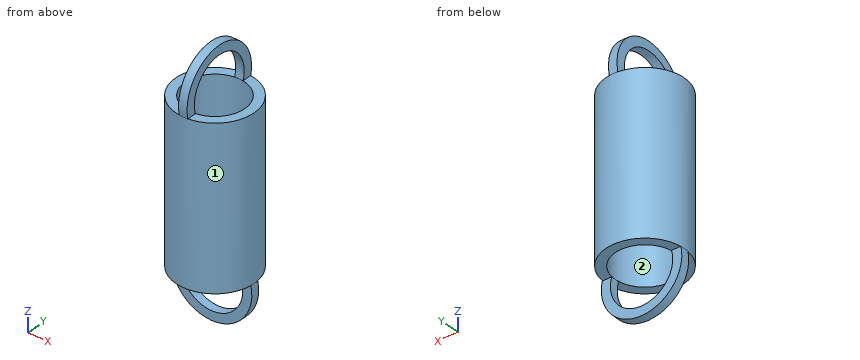
from build123d import *

# Parameters (mm, degrees)
SKETCH1_R           = 4.6
SKETCH1_R_2         = 3.5
BOSS_EXTRUDE1_DEPTH = 9.35
BOSS_EXTRUDE2_DEPTH = 0.5
BOSS_EXTRUDE3_DEPTH = 0.5


with BuildPart() as part:
    # Sketch1 → Boss-Extrude1 (new, symmetric)
    with BuildSketch(Plane.XY):
        Circle(SKETCH1_R)
        Circle(SKETCH1_R_2, mode=Mode.SUBTRACT)
    extrude(amount=BOSS_EXTRUDE1_DEPTH, both=True)

    # Sketch2 → Boss-Extrude2 (add, symmetric)
    with BuildSketch(Plane(origin=(0, 0, 0), x_dir=(0, 0, -1), z_dir=(1, 0, 0))):
        with BuildLine():
            Line((-9.35, -4.6), (-9.35, -3.5))
            ThreePointArc((-9.35, -3.5), (-13.990054945, 0), (-9.35, 3.5))
            Line((-9.35, 3.5), (-9.35, 4.6))
            ThreePointArc((-9.35, 4.6), (-15.057440918, 0), (-9.35, -4.6))
        make_face()
    extrude(amount=BOSS_EXTRUDE2_DEPTH, both=True)

    # Sketch4 → Boss-Extrude3 (add, symmetric)
    with BuildSketch(Plane(origin=(0, 0, 0), x_dir=(1, 0, 0), z_dir=(0, 1, 0))):
        with BuildLine():
            Line((4.6, 9.35), (3.5, 9.35))
            ThreePointArc((3.5, 9.35), (0, 13.990054945), (-3.5, 9.35))
            Line((-3.5, 9.35), (-4.6, 9.35))
            ThreePointArc((-4.6, 9.35), (0, 15.057440918), (4.6, 9.35))
        make_face()
    extrude(amount=BOSS_EXTRUDE3_DEPTH, both=True)


solid = part.part
For this review, take the finished solid that the model builds, in its own axes (mm). Face numbers are marked on the shaded views. Coordinates: 2 decimals unless noted, no trailing zeros. Loops run counter-clockwise (first coordinate to the right, second up) from the corner with the lowest first, then second, coordinate; pieces in that order, holes last. Notation, with made-up numbers: (18, 39) - (30, 39) arc R27 ccw to (30, 68) - close; hole circle Ø5 at (56.25, 60.25). An arc over 180 degrees is marked (long way). Use a Markdown table: item, result. Add a question column.
Item 1: We need section A-A (z = -10.35). Give the boundary of the cut face in (x, y), and give its area (3 significant figures).
Item 2: For line 1 (Z direction, x = 0, y = -0.1); line 2 (X direction, y = 0, z = -1.75); line 3 (Y direction, x = 0.2, z = 10.35), list the stretches that pass through material, from the lowest coordinate up.
Item 3: Insertion check: pin 1 Ø3 at (y, z) = (-2, -8.5) entering from -X; pin 2 Ø1.4 at (x, y) = (0, 1.5) entering from -Z; pin 3 Ø3 at (x, z) = (0, -13) entering from +Y; pin 4 Ø1.7 at (x, z) = (1, -11.5) entering from -Y. Each pin has a flat end and moves straight along its axis. Give the tip position at first contact, or say it passes through.
Item 4: We need section B-B (y = 1.75). Give the boundary of the cut face in (x, z), and give its area (3 significant figures).
Item 5: Mouldability with a two-part tool opening along X and no side actions: class the marked faces 1 and 2 as pulls with the +X half, pulls with the -X half, needs draft (parallel to the pull), parting line crosses it, or undercut.
Item 6: We need section C-C (x = -1.5). Give the boundary of the cut face in (y, z).
Item 7: We need section D-D (z = 7.5). Give the boundary of the cut face in (x, y), and give its area (3 significant figures).
Results list:
| question | item | result |
|---|---|---|
| 1 | outline | (-4.71, -0.5) - (-3.64, -0.5) - (-3.64, 0.5) - (-4.71, 0.5) - close; (3.64, -0.5) - (4.71, -0.5) - (4.71, 0.5) - (3.64, 0.5) - close |
| 1 | area | 2.13 mm^2 |
| 2 | line 1 | z = -15.06 to -13.99, 13.99 to 15.06 |
| 2 | line 2 | x = -4.6 to -3.5, 3.5 to 4.6 |
| 2 | line 3 | y = -4.71 to -3.64, 3.64 to 4.71 |
| 3 | pin 1 | stops at x = -4.57 |
| 3 | pin 2 | stops at z = 13.25 |
| 3 | pin 3 | stops at y = 0.5 |
| 3 | pin 4 | passes through |
| 4 | outline | (-4.25, -9.35) - (-3.03, -9.35) - (-3.03, 9.35) - (-4.25, 9.35) - close; (-0.5, 13.54) - (0.5, 13.54) - (0.5, 14.72) - (-0.5, 14.72) - close; (3.03, -9.35) - (4.25, -9.35) - (4.25, 9.35) - (3.03, 9.35) - close |
| 4 | area | 46.9 mm^2 |
| 5 | face 1 | parting line crosses it |
| 5 | face 2 | undercut |
| 6 | outline | (-4.35, -9.35) - (-3.16, -9.35) - (-3.16, 9.35) - (-4.35, 9.35) - close; (-0.5, -14.81) - (0.5, -14.81) - (0.5, -13.67) - (-0.5, -13.67) - close; (3.16, -9.35) - (4.35, -9.35) - (4.35, 9.35) - (3.16, 9.35) - close |
| 7 | outline | circle Ø9.2 at (0, 0); hole circle Ø7 at (0, 0) |
| 7 | area | 28.0 mm^2 |
